from build123d import *

# Parameters (mm, degrees)
F0_R     = 2.5
F1_DEPTH = 45
F2_W     = 0.7
F2_H     = 0.5
F5_R     = 1
F6_DEPTH = 12.5
F7_R     = 0.25


with BuildPart() as f1:
    # F0 (on Front) → F1 (new body, symmetric)
    with BuildSketch(Plane.XZ):
        Circle(F0_R)
    extrude(amount=F1_DEPTH, both=True)

    # F2 (on Right) → F4 (revolve, cut)
    with BuildSketch(Plane.YZ):
        with Locations((-30.65, 2.25)):
            Rectangle(F2_W, F2_H)
        with Locations((30.65, 2.25)):
            Rectangle(F2_W, F2_H)
    revolve(axis=Axis((0, -3.298404, 0), (0, 1, 0)), mode=Mode.SUBTRACT)

    # F5 (on Right) → F6 (cut, symmetric)
    with BuildSketch(Plane.YZ):
        with Locations((-43, 0)):
            Circle(F5_R)
        with Locations((43, 0)):
            Circle(F5_R)
        Circle(F5_R)
    extrude(amount=F6_DEPTH, both=True, mode=Mode.SUBTRACT)

    # F7
    f7_edges = [f1.edges().sort_by_distance(p)[0] for p in [
        (0, -31, -2),
        (0, -30.3, -2),
        (0, 30.3, -2),
        (0, 31, -2),
    ]]
    fillet(f7_edges, radius=F7_R)


solid = f1.part
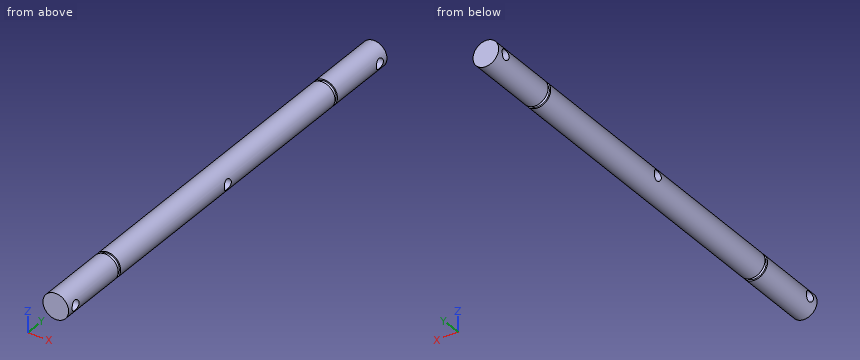
Can you work these out from the model? Positions are in its coordinate system, mm. Coordinates: 2 decimals unless noted, no trailing zeros. Write each loop counter-clockwise with the first axis right and the second up, starting at its lowest first coordinate (ties: lowest second). Pieces come first, ordered by that corner, then holes. Notation, with made-up numbers: (26.5, 3) - (73.5, 3) arc R30 cw to (73.5, 27) - close; hole circle Ø10 at (9.5, 21). An arc over 180 degrees is marked (long way). Return JSON: item names as keys, results as strings. Group by question number.
Item 1: If we section it at B-B (y = 0): Write out the boundary of the cut face in (x, z), then the cut area to 3 significant figures.
Item 2: I'm going to push a flat-ended pin straight in: pin 1 Ø1.2 at (y, z) = (43, 0) entering from +X. Where does the tip first touch, or does it pass through?
Item 3: If we section it at A-A (y = -27): Write out the boundary of the cut face in (x, z), then the cut area to 3 significant figures.
Item 4: Please list where these lines run through material, in increasing order: probe 1 along Y at (x, z) = (1.3, 0); probe 2 along Y at (x, z) = (-1.8, -1.35); probe 3 along Z at (x, y) = (0, 0).
Return value:
{
 "1": {"outline": "(-2.29, -1) arc R2.5 ccw to (2.29, -1) - close; (-2.29, 1) - (2.29, 1) arc R2.5 ccw to start", "area": "9.91 mm^2"},
 "2": {"pin 1": "passes through"},
 "3": {"outline": "circle Ø5 at (0, 0)", "area": "19.6 mm^2"},
 "4": {"probe 1": "y = -45 to -44, -42 to -1, 1 to 42, 44 to 45", "probe 2": "y = -45 to -31, -30.3 to 30.3, 31 to 45", "probe 3": "z = -2.5 to -1, 1 to 2.5"}
}
